from build123d import *

# Parameters (mm, degrees)
F0_W          = 30
F0_H          = 16
F1_DEPTH      = 1.28
F3_DEPTH      = 3.75
F5_DEPTH      = 2.8
F7_DEPTH      = 3.75
F8_W          = 2.9444776119
F8_H          = 5.2
F9_DEPTH      = 0.68
F10_T1_DEPTH  = 7.5
F10_T6_DEPTH  = 20.75
F10_T11_DEPTH = 24.5
F10_T16_DEPTH = 20.75
F10_T21_DEPTH = 24.5
F10_T26_DEPTH = 9.5055223881
F10_T31_DEPTH = 5.7555223881
F10_T36_DEPTH = 9.5055223881
F10_T41_DEPTH = 5.7555223881
F10_T47_DEPTH = 8.9958162388
F10_T51_DEPTH = 20.75
F10_T59_DEPTH = 20.75
F10_T64_DEPTH = 8.9958162388
F10_T71_DEPTH = 9.5055223881
F10_T76_DEPTH = 11.25
F10_T83_DEPTH = 11.25
F10_T87_DEPTH = 9.5055223881
F11_R         = 2.8
F12_DEPTH     = 1.3
F14_DEPTH     = 2.5


# Not quite as in the source:
# - a fillet or chamfer that OpenCascade refuses, or shapes differently, is made with other operations: its cross-section is extruded or revolved along the edge and cut away or added


with BuildPart() as f1:
    # F0 (on Top) → F1 (new body)
    with BuildSketch(Plane.XY):
        with Locations((1.94, 0)):
            Rectangle(F0_W, F0_H)
    extrude(amount=F1_DEPTH)

    # F2 (on Front) → F3 (join, symmetric)
    with BuildSketch(Plane.XZ):
        Polygon((5.24, 4.98), (-7.86, 4.98), (-11.76, 1.28), (5.24, 1.28), align=None)
    extrude(amount=F3_DEPTH, both=True)

    # F4 (on Front) → F5 (join, symmetric)
    with BuildSketch(Plane.XZ):
        Polygon((13.94, 10.5), (5.24, 4.48), (5.24, -1.6), (12.09, 5.1), (13.94, 5.1), align=None)
    extrude(amount=F5_DEPTH, both=True)

    # F6 (on Front) → F7 (join, symmetric)
    with BuildSketch(Plane.XZ):
        Polygon((13.94, 5.1), (12.09, 5.1), (6.8758208955, 0), (13.94, 0), align=None)
    extrude(amount=F7_DEPTH, both=True)

    # F8 (on face) → F9 (join)
    with BuildSketch(Plane.XY.offset(1.28)):
        with Locations((6.712238806, -5.4)):
            Rectangle(F8_W, F8_H)
        with Locations((6.712238806, 5.4)):
            Rectangle(F8_W, F8_H)
    extrude(amount=F9_DEPTH)

    # F10: fillet of radius 1.5 on 6 edges, made by hand

    # F10_s2 → F10_t1 (join)
    with BuildSketch(Plane.XZ.offset(-3.75)):
        with BuildLine():
            ThreePointArc((15.44, 1.28), (14.3793398282, 1.7193398282), (13.94, 2.78))
            Line((13.94, 2.78), (13.94, 1.28))
            Line((13.94, 1.28), (15.44, 1.28))
        make_face()
        with BuildLine():
            ThreePointArc((-12.3583264955, 1.28), (-11.802580745, 1.3867496058), (-11.3259358476, 1.6918044522))
            Line((-11.3259358476, 1.6918044522), (-11.76, 1.28))
            Line((-11.76, 1.28), (-12.3583264955, 1.28))
        make_face()
    extrude(amount=F10_T1_DEPTH)


with BuildPart() as f10_tool4:
    # F10_s5 → F10_t6 (new body)
    with BuildSketch(Plane.YZ.offset(-15.51)):
        with BuildLine():
            ThreePointArc((-5.25, 1.28), (-4.1893398282, 1.7193398282), (-3.75, 2.78))
            Line((-3.75, 2.78), (-3.75, 1.28))
            Line((-3.75, 1.28), (-5.25, 1.28))
        make_face()
    extrude(amount=F10_T6_DEPTH)

    split(bisect_by=Plane(origin=(-6.2098546713, 0, 6.5455224913), x_dir=(0, 1, 0), z_dir=(0.6882604319, 0, -0.7254636985)), keep=Keep.TOP)


with BuildPart() as f1_1:
    add(f1.part)

    # F10_t3: union F10_tool4
    add(f10_tool4.part)


with BuildPart() as f10_tool9:
    # F10_s10 → F10_t11 (new body)
    with BuildSketch(Plane.YZ.offset(-15.51)):
        with BuildLine():
            ThreePointArc((-5.25, 1.28), (-4.1893398282, 1.7193398282), (-3.75, 2.78))
            Line((-3.75, 2.78), (-3.75, 1.28))
            Line((-3.75, 1.28), (-5.25, 1.28))
        make_face()
    extrude(amount=F10_T11_DEPTH)

    split(bisect_by=Plane(origin=(3.361803676, 0, -3.4370679374), x_dir=(0, 1, 0), z_dir=(0.6992361874, 0, -0.7148907289)), keep=Keep.TOP)


with BuildPart() as f1_2:
    add(f1_1.part)

    # F10_t8: union F10_tool9
    add(f10_tool9.part)


with BuildPart() as f10_tool14:
    # F10_s15 → F10_t16 (new body)
    with BuildSketch(Plane.YZ.offset(-15.51)):
        with BuildLine():
            ThreePointArc((5.25, 1.28), (4.1893398282, 1.7193398282), (3.75, 2.78))
            Line((3.75, 2.78), (3.75, 1.28))
            Line((3.75, 1.28), (5.25, 1.28))
        make_face()
    extrude(amount=F10_T16_DEPTH)

    split(bisect_by=Plane(origin=(-6.2098546713, 0, 6.5455224913), x_dir=(0, 1, 0), z_dir=(0.6882604319, 0, -0.7254636985)), keep=Keep.TOP)


with BuildPart() as f1_3:
    add(f1_2.part)

    # F10_t13: union F10_tool14
    add(f10_tool14.part)


with BuildPart() as f10_tool19:
    # F10_s20 → F10_t21 (new body)
    with BuildSketch(Plane.YZ.offset(-15.51)):
        with BuildLine():
            ThreePointArc((5.25, 1.28), (4.1893398282, 1.7193398282), (3.75, 2.78))
            Line((3.75, 2.78), (3.75, 1.28))
            Line((3.75, 1.28), (5.25, 1.28))
        make_face()
    extrude(amount=F10_T21_DEPTH)

    split(bisect_by=Plane(origin=(3.361803676, 0, -3.4370679374), x_dir=(0, 1, 0), z_dir=(0.6992361874, 0, -0.7148907289)), keep=Keep.TOP)


with BuildPart() as f1_4:
    add(f1_3.part)

    # F10_t18: union F10_tool19
    add(f10_tool19.part)


with BuildPart() as f10_tool24:
    # F10_s25 → F10_t26 (new body)
    with BuildSketch(Plane.YZ.offset(4.4344776119)):
        with BuildLine():
            ThreePointArc((-5.25, 1.28), (-4.1893398282, 1.7193398282), (-3.75, 2.78))
            Line((-3.75, 2.78), (-3.75, 1.28))
            Line((-3.75, 1.28), (-5.25, 1.28))
        make_face()
    extrude(amount=F10_T26_DEPTH)

    split(bisect_by=Plane.YZ.offset(5.24), keep=Keep.BOTTOM)


with BuildPart() as f1_5:
    add(f1_4.part)

    # F10_t23: union F10_tool24
    add(f10_tool24.part)


with BuildPart() as f10_tool29:
    # F10_s30 → F10_t31 (new body)
    with BuildSketch(Plane.YZ.offset(8.1844776119)):
        with BuildLine():
            ThreePointArc((-5.25, 1.28), (-4.1893398282, 1.7193398282), (-3.75, 2.78))
            Line((-3.75, 2.78), (-3.75, 1.28))
            Line((-3.75, 1.28), (-5.25, 1.28))
        make_face()
    extrude(amount=F10_T31_DEPTH)

    split(bisect_by=Plane(origin=(3.361803676, 0, -3.4370679374), x_dir=(0, 1, 0), z_dir=(0.6992361874, 0, -0.7148907289)), keep=Keep.TOP)


with BuildPart() as f1_6:
    add(f1_5.part)

    # F10_t28: union F10_tool29
    add(f10_tool29.part)


with BuildPart() as f10_tool34:
    # F10_s35 → F10_t36 (new body)
    with BuildSketch(Plane.YZ.offset(4.4344776119)):
        with BuildLine():
            ThreePointArc((5.25, 1.28), (4.1893398282, 1.7193398282), (3.75, 2.78))
            Line((3.75, 2.78), (3.75, 1.28))
            Line((3.75, 1.28), (5.25, 1.28))
        make_face()
    extrude(amount=F10_T36_DEPTH)

    split(bisect_by=Plane.YZ.offset(5.24), keep=Keep.BOTTOM)


with BuildPart() as f1_7:
    add(f1_6.part)

    # F10_t33: union F10_tool34
    add(f10_tool34.part)


with BuildPart() as f10_tool39:
    # F10_s40 → F10_t41 (new body)
    with BuildSketch(Plane.YZ.offset(8.1844776119)):
        with BuildLine():
            ThreePointArc((5.25, 1.28), (4.1893398282, 1.7193398282), (3.75, 2.78))
            Line((3.75, 2.78), (3.75, 1.28))
            Line((3.75, 1.28), (5.25, 1.28))
        make_face()
    extrude(amount=F10_T41_DEPTH)

    split(bisect_by=Plane(origin=(3.361803676, 0, -3.4370679374), x_dir=(0, 1, 0), z_dir=(0.6992361874, 0, -0.7148907289)), keep=Keep.TOP)


with BuildPart() as f1_8:
    add(f1_7.part)

    # F10_t38: union F10_tool39
    add(f10_tool39.part)


with BuildPart() as f10_tool45:
    # F10_s46 → F10_t47 (new body)
    with BuildSketch(Plane.XZ.offset(-3.75)):
        with BuildLine():
            ThreePointArc((-12.3583264955, 1.28), (-11.802580745, 1.3867496058), (-11.3259358476, 1.6918044522))
            Line((-11.3259358476, 1.6918044522), (-11.76, 1.28))
            Line((-11.76, 1.28), (-12.3583264955, 1.28))
        make_face()
    extrude(amount=F10_T47_DEPTH)

    split(bisect_by=Plane.XZ.offset(3.75), keep=Keep.TOP)


with BuildPart() as f10_tool49:
    # F10_s50 → F10_t51 (new body)
    with BuildSketch(Plane.YZ.offset(-15.51)):
        with BuildLine():
            ThreePointArc((-5.25, 1.28), (-4.1893398282, 1.7193398282), (-3.75, 2.78))
            Line((-3.75, 2.78), (-3.75, 1.28))
            Line((-3.75, 1.28), (-5.25, 1.28))
        make_face()
    extrude(amount=F10_T51_DEPTH)

    split(bisect_by=Plane.YZ.offset(-13.06), keep=Keep.TOP)

    split(bisect_by=Plane(origin=(-6.2098546713, 0, 6.5455224913), x_dir=(0, 1, 0), z_dir=(-0.6882604319, 0, 0.7254636985)), keep=Keep.TOP)


with BuildPart() as f10_tool45_1:
    add(f10_tool45.part)

    # F10_t54: intersect F10_tool49
    add(f10_tool49.part, mode=Mode.INTERSECT)


with BuildPart() as f1_9:
    add(f1_8.part)

    # F10_t43: union F10_tool45
    add(f10_tool45_1.part)


with BuildPart() as f10_tool57:
    # F10_s58 → F10_t59 (new body)
    with BuildSketch(Plane.YZ.offset(-15.51)):
        with BuildLine():
            ThreePointArc((5.25, 1.28), (4.1893398282, 1.7193398282), (3.75, 2.78))
            Line((3.75, 2.78), (3.75, 1.28))
            Line((3.75, 1.28), (5.25, 1.28))
        make_face()
    extrude(amount=F10_T59_DEPTH)

    split(bisect_by=Plane.YZ.offset(-13.06), keep=Keep.TOP)

    split(bisect_by=Plane(origin=(-6.2098546713, 0, 6.5455224913), x_dir=(0, 1, 0), z_dir=(-0.6882604319, 0, 0.7254636985)), keep=Keep.TOP)


with BuildPart() as f10_tool62:
    # F10_s63 → F10_t64 (new body)
    with BuildSketch(Plane.XZ.offset(-5.2458162388)):
        with BuildLine():
            ThreePointArc((-12.3583264955, 1.28), (-11.802580745, 1.3867496058), (-11.3259358476, 1.6918044522))
            Line((-11.3259358476, 1.6918044522), (-11.76, 1.28))
            Line((-11.76, 1.28), (-12.3583264955, 1.28))
        make_face()
    extrude(amount=F10_T64_DEPTH)

    split(bisect_by=Plane.XZ.offset(-3.75), keep=Keep.BOTTOM)


with BuildPart() as f10_tool57_1:
    add(f10_tool57.part)

    # F10_t66: intersect F10_tool62
    add(f10_tool62.part, mode=Mode.INTERSECT)


with BuildPart() as f1_10:
    add(f1_9.part)

    # F10_t55: union F10_tool57
    add(f10_tool57_1.part)


with BuildPart() as f10_tool69:
    # F10_s70 → F10_t71 (new body)
    with BuildSketch(Plane.YZ.offset(8.1844776119)):
        with BuildLine():
            ThreePointArc((-5.25, 1.28), (-4.1893398282, 1.7193398282), (-3.75, 2.78))
            Line((-3.75, 2.78), (-3.75, 1.28))
            Line((-3.75, 1.28), (-5.25, 1.28))
        make_face()
    extrude(amount=F10_T71_DEPTH)

    split(bisect_by=Plane.YZ.offset(16.94), keep=Keep.BOTTOM)

    split(bisect_by=Plane.YZ.offset(13.94), keep=Keep.TOP)


with BuildPart() as f10_tool74:
    # F10_s75 → F10_t76 (new body)
    with BuildSketch(Plane.XZ.offset(7.5)):
        with BuildLine():
            ThreePointArc((15.44, 1.28), (14.3793398282, 1.7193398282), (13.94, 2.78))
            Line((13.94, 2.78), (13.94, 1.28))
            Line((13.94, 1.28), (15.44, 1.28))
        make_face()
    extrude(amount=-F10_T76_DEPTH)

    split(bisect_by=Plane.XZ.offset(3.75), keep=Keep.TOP)


with BuildPart() as f10_tool69_1:
    add(f10_tool69.part)

    # F10_t78: intersect F10_tool74
    add(f10_tool74.part, mode=Mode.INTERSECT)


with BuildPart() as f1_11:
    add(f1_10.part)

    # F10_t67: union F10_tool69
    add(f10_tool69_1.part)


with BuildPart() as f10_tool81:
    # F10_s82 → F10_t83 (new body)
    with BuildSketch(Plane.XZ.offset(3.75)):
        with BuildLine():
            ThreePointArc((15.44, 1.28), (14.3793398282, 1.7193398282), (13.94, 2.78))
            Line((13.94, 2.78), (13.94, 1.28))
            Line((13.94, 1.28), (15.44, 1.28))
        make_face()
    extrude(amount=-F10_T83_DEPTH)

    split(bisect_by=Plane.XZ.offset(-3.75), keep=Keep.BOTTOM)


with BuildPart() as f10_tool85:
    # F10_s86 → F10_t87 (new body)
    with BuildSketch(Plane.YZ.offset(8.1844776119)):
        with BuildLine():
            ThreePointArc((5.25, 1.28), (4.1893398282, 1.7193398282), (3.75, 2.78))
            Line((3.75, 2.78), (3.75, 1.28))
            Line((3.75, 1.28), (5.25, 1.28))
        make_face()
    extrude(amount=F10_T87_DEPTH)

    split(bisect_by=Plane.YZ.offset(16.94), keep=Keep.BOTTOM)

    split(bisect_by=Plane.YZ.offset(13.94), keep=Keep.TOP)


with BuildPart() as f10_tool81_1:
    add(f10_tool81.part)

    # F10_t90: intersect F10_tool85
    add(f10_tool85.part, mode=Mode.INTERSECT)


with BuildPart() as f1_12:
    add(f1_11.part)

    # F10_t79: union F10_tool81
    add(f10_tool81_1.part)

    # F11 (on face) → F12 (cut)
    with BuildSketch(Plane.XY.offset(4.98)):
        Circle(F11_R)
    extrude(amount=-F12_DEPTH, mode=Mode.SUBTRACT)

    # F13 (on Front) → F14 (cut, symmetric)
    with BuildSketch(Plane.XZ):
        Polygon((-6.56, 3.9), (-10.56, 0), (5.24, 0), (5.24, 3.9), (3.41, 3.9), (1.75, 1.8), (-1.75, 1.8), (-3.41, 3.9), align=None)
        Polygon((11.8855223881, 4.9), (6.8758208955, 0), (13.54, 0), (13.316296041, 4.9), align=None)
    extrude(amount=F14_DEPTH, both=True, mode=Mode.SUBTRACT)

    # F15 (on Front) → F16 (revolve)
    with BuildSketch(Plane.XZ):
        with BuildLine():
            Line((13.94, 7.8), (14.5818286702, 7.8))
            ThreePointArc((14.5818286702, 7.8), (14.4191665899, 9.1876188275), (13.94, 10.5))
            Line((13.94, 10.5), (13.94, 7.8))
        make_face()
    revolve(axis=Axis((14.2609143351, 0, 7.8), (1, 0, 0)))


solid = f1_12.part
For this review, take the finished solid that the model builds, in its own axes (mm). A direction names the side the tool comes from. Round coordinates to 2 decimals unless told otherwise and drop trailing zeros. Loops run counter-clockwise (first coordinate to the right, second up) from the corner with the lowest first, then second, coordinate; pieces in that order, holes last. Notation, with made-up numbers: (2, -27.5) - (11, -27.5) arc R24 ccw to (11, 2.5) - close; hole circle Ø4 at (-26.75, 22). An arc over 180 degrees is marked (long way). Put each result on its own line as item: value. Start each with the question number.
1. For probe 1 along Y at (x, z) = (0, 4.3); probe 2 along Z at (x, y) = (5, 3.25); probe 3 along Y at (x, z) = (9.5, 0.25), list the stretches that pass through material, from the lowest coordinate up. Write a range as [from, to].
2. Consider section D-D on x = 7.5. State the section outline as (y, z) points, plus the area to 3 significant figures.
3. Consider section C-C on z = 9.25. State the section outline as (x, y) points.
4. Consider section B-B on x = 0. State the section outline as (y, z) points, plus the area to 3 significant figures.
5. Mouldability with a two-part tool opening along Z and no side actions: class faces 1 (the cylindrical face through (-3.68, -4.2, 1.71)), 2 (the flat face through (12, -3.75, 4)), 3 (the cylindrical face through (14.4, -0.1, 1.7)) as +Z half, -Z half, draft (parallel to the pull), parting line (faces both ways), or undercut.
6. For faces 4 (the flat face through (0, 0, 3.68)), 5 (the cylindrical face through (11.76, -4.2, 1.71)), 6 (the flat face through (13, 3, 5.1)), list the 3-axis set-ups (+Z, -Z, +X, -X, +Y, -Y) from which the entire face can be reached by the end or side of a thin tool; tool diameter is ignored.
7. Consider section A-A on y = 6.75. State the section outline as (x, z) points, plus the area to 3 significant figures.
8. Insertion check: P1, Ø0.9, axis at y = 0, z = 3, coming from the +X side; P2, Ø1.8, axis at x = -0.5, z = 3.5, coming from the +Y side; P3, Ø8, axis at x = 11, y = 0.5, coming from the -Z side; P4, Ø2, axis at y = 4.5, z = 9, coming from the -X side. Each pin has a flat end and moves straight along its axis. Give the tip position at first contact, or say it passes through.
Result sheet:
1. probe 1: [-3.75, -2.8], [2.8, 3.75]
1. probe 2: [0, 4.98]
1. probe 3: [-8, -2.5], [2.5, 8]
2. outline: (-8, 0) - (-2.5, 0) - (-2.5, 0.61) - (2.5, 0.61) - (2.5, 0) - (8, 0) - (8, 1.96) - (2.8, 1.96) - (2.8, 6.04) - (-2.8, 6.04) - (-2.8, 1.96) - (-8, 1.96) - close
2. area: 51.2 mm^2
3. outline: (12.13, -2.8) - (13.94, -2.8) - (13.94, -2.28) arc R5.82 ccw to (13.94, 2.28) - (13.94, 2.8) - (12.13, 2.8) - close
4. outline: (-8, 0) - (-2.5, 0) - (-2.5, 1.8) - (2.5, 1.8) - (2.5, 0) - (8, 0) - (8, 1.28) - (5.25, 1.28) arc R1.5 cw to (3.75, 2.78) - (3.75, 4.98) - (2.8, 4.98) - (2.8, 3.68) - (-2.8, 3.68) - (-2.8, 4.98) - (-3.75, 4.98) - (-3.75, 2.78) arc R1.5 cw to (-5.25, 1.28) - (-8, 1.28) - close
4. area: 32.9 mm^2
5. face 1: +Z half
5. face 2: draft
5. face 3: undercut
6. face 4: +Z
6. face 5: +Z, +X, -Y
6. face 6: +Z, +X, -X, +Y
7. outline: (-13.06, 0) - (16.94, 0) - (16.94, 1.28) - (8.18, 1.28) - (8.18, 1.96) - (5.24, 1.96) - (5.24, 1.28) - (-13.06, 1.28) - close
7. area: 40.4 mm^2
8. P1: x = 13.96
8. P2: y = 3.76
8. P3: z = 0
8. P4: through
